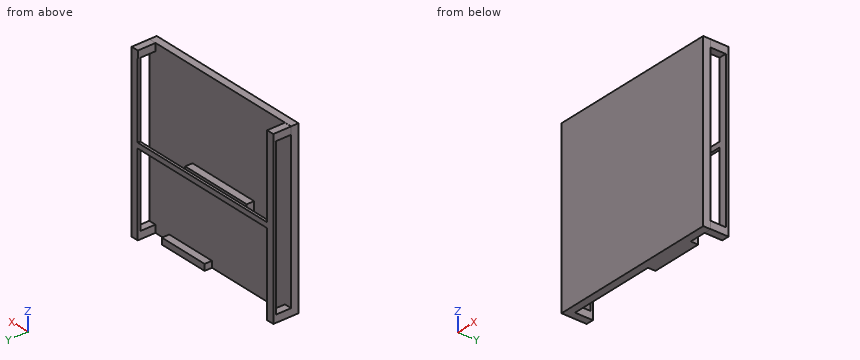
from build123d import *

# Parameters (mm, degrees)
SKETCH1_W            = 115
SKETCH1_H            = 115
BOSS_EXTRUDE3_DEPTH  = 5
SKETCH5_W            = 50
SKETCH5_H            = 6
SKETCH5_W_2          = 34.678216068
SKETCH5_H_2          = 4.225459606
BOSS_EXTRUDE4_DEPTH  = 5
SKETCH6_W            = 5
SKETCH6_H            = 5
BOSS_EXTRUDE5_DEPTH  = 12
SKETCH8_W            = 5
SKETCH8_H            = 1.75
BOSS_EXTRUDE7_DEPTH  = 105
SKETCH9_W            = 5
SKETCH9_H            = 1.75
BOSS_EXTRUDE8_DEPTH  = 105
SKETCH11_W           = 3.5
SKETCH11_H           = 1.75
BOSS_EXTRUDE10_DEPTH = 108


with BuildPart() as part:
    # Sketch1 → Boss-Extrude3 (new body)
    with BuildSketch(Plane(origin=(0, 0, 0), x_dir=(1, 0, 0), z_dir=(0, 1, 0))):
        Rectangle(SKETCH1_W, SKETCH1_H)
    extrude(amount=BOSS_EXTRUDE3_DEPTH)

    # Sketch5 → Boss-Extrude4 (add)
    with BuildSketch(Plane(origin=(0, 5, 0), x_dir=(1, 0, 0), z_dir=(0, 1, 0))):
        with Locations((-2.5, 4.5)):
            Rectangle(SKETCH5_W, SKETCH5_H)
        with Locations((24.044261594, 55.387270197)):
            Rectangle(SKETCH5_W_2, SKETCH5_H_2)
    extrude(amount=BOSS_EXTRUDE4_DEPTH)

    # Sketch6 → Boss-Extrude5 (add)
    with BuildSketch(Plane(origin=(0, 5, 0), x_dir=(1, 0, 0), z_dir=(0, 1, 0))):
        with Locations((-55.003212796, -54.936396199)):
            Rectangle(SKETCH6_W, SKETCH6_H)
        with Locations((-55, 55)):
            Rectangle(SKETCH6_W, SKETCH6_H)
        with Locations((55.107980821, 54.950828784)):
            Rectangle(SKETCH6_W, SKETCH6_H)
        with Locations((54.988780211, -55.003212796)):
            Rectangle(SKETCH6_W, SKETCH6_H)
    extrude(amount=BOSS_EXTRUDE5_DEPTH)

    # Sketch8 → Boss-Extrude7 (add)
    with BuildSketch(Plane.XY.offset(-52.5)):
        with Locations((-55, 16.125)):
            Rectangle(SKETCH8_W, SKETCH8_H)
    extrude(amount=BOSS_EXTRUDE7_DEPTH)

    # Sketch9 → Boss-Extrude8 (add)
    with BuildSketch(Plane.XY.offset(-52.450828784)):
        with Locations((55.107980821, 16.125)):
            Rectangle(SKETCH9_W, SKETCH9_H)
    extrude(amount=BOSS_EXTRUDE8_DEPTH)

    # Sketch11 → Boss-Extrude10 (add)
    with BuildSketch(Plane(origin=(-52.5, 0, 0), x_dir=(0, 0, -1), z_dir=(1, 0, 0))):
        with Locations((0.033603801, 16.125)):
            Rectangle(SKETCH11_W, SKETCH11_H)
    extrude(amount=BOSS_EXTRUDE10_DEPTH)


solid = part.part
Geometry: final body of the model. Coordinates: model frame, mm. Round coordinates to 2 decimals unless told otherwise and drop trailing zeros. Loops run counter-clockwise (first coordinate to the right, second up) from the corner with the lowest first, then second, coordinate; pieces in that order, holes last.
Q1. Section D-D on x = 28.5. Return loops of the section in (y, z).
Q2. Section A-A on x = -14.5. Return loops of the section in (y, z), plus the area to 3 significant figures.
Q3. Pin query (flat end, axial travel): P1, Ø4, axis at x = -41.5, z = 27, coming from the +Y side; P2, Ø1.5, axis at x = -56, y = 12, coming from the +Z side; P3, Ø2, axis at y = 7.5, z = -55, coming from the -X side. Return the tip coordinate at first contact, or that it passes through.
Q4. Section C-C on y = 7. Return loops of the section in (x, z), plus the area to 3 significant figures.
Q5. Material intervals for L1, parallel to X at y = 16.5, z = -42; L2, parallel to X at y = 4.25, z = 40; L3, parallel to Y at x = -49, z = -34, sorted ascending.
Q6. Section B-B on z = -4. Return loops of the section in (x, y), plus the area to 4 significant figures.
Evaluation:
1. outline: (0, -57.5) - (10, -57.5) - (10, -53.27) - (5, -53.27) - (5, 57.5) - (0, 57.5) - close; (15.25, -1.78) - (17, -1.78) - (17, 1.72) - (15.25, 1.72) - close
2. outline: (0, -57.5) - (5, -57.5) - (5, -7.5) - (10, -7.5) - (10, -1.5) - (5, -1.5) - (5, 57.5) - (0, 57.5) - close; (15.25, -1.78) - (17, -1.78) - (17, 1.72) - (15.25, 1.72) - close
2. area: 611 mm2
3. P1: stops at y = 5
3. P2: stops at z = 57.44
3. P3: stops at x = -57.5
4. outline: (-57.5, -57.5) - (-52.5, -57.5) - (-52.5, -52.5) - (-57.5, -52.5) - close; (-57.5, 52.44) - (-52.5, 52.44) - (-52.5, 57.44) - (-57.5, 57.44) - close; (-27.5, -7.5) - (22.5, -7.5) - (22.5, -1.5) - (-27.5, -1.5) - close; (6.71, -57.5) - (41.38, -57.5) - (41.38, -53.27) - (6.71, -53.27) - close; (52.49, 52.5) - (57.49, 52.5) - (57.49, 57.5) - (52.49, 57.5) - close; (52.61, -57.45) - (57.61, -57.45) - (57.61, -52.45) - (52.61, -52.45) - close
4. area: 547 mm2
5. L1: x = -57.5 to -52.5, 52.61 to 57.61
5. L2: x = -57.5 to 57.5
5. L3: y = 0 to 5
6. outline: (-57.5, 0) - (57.5, 0) - (57.5, 5) - (22.5, 5) - (22.5, 10) - (-27.5, 10) - (-27.5, 5) - (-57.5, 5) - close; (-57.5, 15.25) - (-52.5, 15.25) - (-52.5, 17) - (-57.5, 17) - close; (52.61, 15.25) - (57.61, 15.25) - (57.61, 17) - (52.61, 17) - close
6. area: 842.5 mm2
